from build123d import *

# Parameters (mm, degrees)
SKETCH2_R          = 2.5
CUT_EXTRUDE1_DEPTH = 47.445475819
CIRPATTERN1_COUNT  = 10


with BuildPart() as part:
    # Sketch1 → Revolve1 (revolve)
    with BuildSketch(Plane.XY, mode=Mode.PRIVATE) as revolve1_sk:
        Polygon((-5, 0), (5, 0), (5, -4), (12, -4), (16.497946055, -15.125128372), (13, -20), (-13, -20), (-16.497946055, -15.125128372), (-12, -4), (-5, -4), align=None)
    revolve(revolve1_sk.sketch.rotate(Axis((0, 7, 0), (1, 0, 0)), 270), axis=Axis((0, 7, 0), (1, 0, 0)))

    # SurfaceCut1
    split(bisect_by=Plane(origin=(0, 0, 0), x_dir=(0, 0, -1), z_dir=(1, 0, 0)), keep=Keep.TOP)

    # SurfaceCut4
    split(bisect_by=Plane(origin=(12, 0, 0), x_dir=(0, 0, -1), z_dir=(1, 0, 0)), keep=Keep.BOTTOM)

    # Sketch2 → Cut-Extrude1 (cut, through all)
    with BuildSketch(Plane(origin=(16.497946055, 0, 0), x_dir=(0, 0, -1), z_dir=(1, 0, 0))):
        with Locations((0, 25.5)):
            Circle(SKETCH2_R)
        with Locations((6, 27.5)):
            Circle(SKETCH2_R)
    extrude(amount=-CUT_EXTRUDE1_DEPTH, mode=Mode.SUBTRACT)

    # CirPattern1: part ×10 about axis
    cirpattern1_axis = Axis((0, 7, 0), (1, 0, 0))


with BuildPart() as part_1:
    add(part.part)
    for i in range(1, CIRPATTERN1_COUNT):
        add(part.part.rotate(cirpattern1_axis, i * 360 / CIRPATTERN1_COUNT))


solid = part_1.part
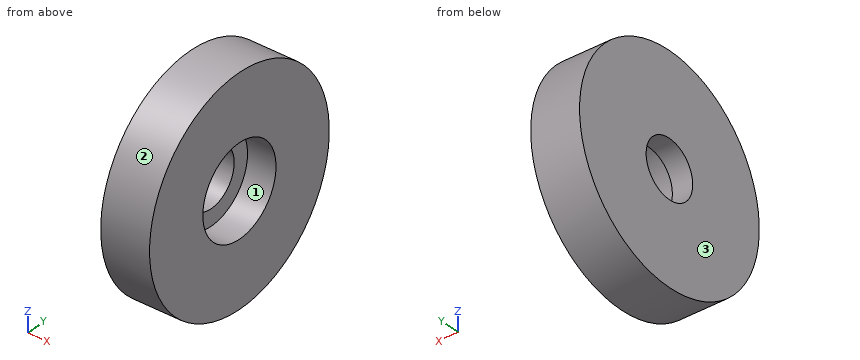
Geometry check sheet. Reference: the model listing, model coordinates, mm. Face numbers are marked on the shaded views. Coordinates: 2 decimals unless noted, no trailing zeros. Order: outer loops, then holes, each group sorted by start corner. A loop starts at its lowest first (then second) coordinate and runs counter-clockwise, first axis right, second up. Notation, with made-up numbers: M 12.25,35.25 L 37.25,35.25 A25 cw 37.25,54.25 Z; hole C -12,61.5 d4. An arc over 180 degrees is marked long. Use CSV: the item, a comma, the result in double quotes.
Item 1: Thickness scan on line 1 along Y through (x, z) = (2.75, 0); line 2 along Y through (x, z) = (9.5, 0); line 3 along Z through (x, y) = (5.5, 13.5). Record the ranges inside material, lowest first.
Returned:
line 1,"y = -20 to 0, 14 to 34"
line 2,"y = -20 to -4, 18 to 34"
line 3,"z = -26.21 to -8.87, 8.87 to 26.21"
Item 2: Mould release check, pull along Z, two halves, no side actions. Record for the marked faces 1, 2 and 3: pulls with the +Z half, pulls with the -Z half, needs draft (parallel to the pull), parting line crosses it, or undercut.
Returned:
face 1,"undercut"
face 2,"parting line crosses it"
face 3,"needs draft"
Item 3: Cross-section at B-B on z = 0. Record the cut outline in (x, y), then the cut area to 3 significant figures.
Returned:
outline,"M 0,-20 L 12,-20 L 12,-4 L 5,-4 L 5,0 L 0,0 Z; M 0,14 L 5,14 L 5,18 L 12,18 L 12,34 L 0,34 Z"
area,"424 mm2"
Item 4: Gauge pin test, flat ends, axial feed: pin 1 Ø20 at (y, z) = (7, 0) entering from +X; pin 2 Ø1.5 at (x, y) = (4, 16.5) entering from +Z; pin 3 Ø5 at (x, z) = (7.5, 9) entering from +Y. Record the tip position at first contact, or that the pin passes through.
Returned:
pin 1,"stops at x = 5"
pin 2,"stops at z = 25.54"
pin 3,"stops at y = 33.21"
Item 5: Cross-section at A-A on y = 7. Record the cut outline in (x, z).
Returned:
outline,"M 0,-27 L 12,-27 L 12,-11 L 5,-11 L 5,-7 L 0,-7 Z; M 0,7 L 5,7 L 5,11 L 12,11 L 12,27 L 0,27 Z"
Item 6: Cross-section at C-C on x = 4.25. Record the cut outline in (y, z), then the cut area to 3 significant figures.
Returned:
outline,"C 7,0 d54; hole C 7,0 d14"
area,"2,140 mm2"
Item 7: Cross-section at D-D on y = -13. Record the cut outline in (x, z).
Returned:
outline,"M 0,-18.14 L 12,-18.14 L 12,18.14 L 0,18.14 Z"
